Can you work these out from the model? Positions are in its coordinate system, mm. A direction names the side the tool comes from. Round coordinates to 2 decimals unless told otherwise and drop trailing zeros. Order: outer loops, then holes, each group sorted by start corner. A loop starts at its lowest first (then second) coordinate and runs counter-clockwise, first axis right, second up.
from build123d import *

# Parameters (mm, degrees)
SKETCH001_W   = 10
SKETCH001_H   = 10
SKETCH001_W_2 = 8
SKETCH001_H_2 = 8
PAD_DEPTH     = 254
SKETCH002_R   = 2.5
POCKET_DEPTH  = 43.001


with BuildPart() as part:
    # Sketch → Revolution (revolve)
    with BuildSketch(Plane.XZ):
        with BuildLine():
            Line((0, 0), (11, 0))
            ThreePointArc((11, 0), (30.091883, 7.908117), (38, 27))
            Line((38, 27), (37, 27))
            ThreePointArc((10.999947, 1), (29.384758, 8.615205), (37, 27))
            Line((10.999947, 1), (0, 1))
            Line((0, 0), (0, 1))
        make_face()
    revolve(axis=Axis((0, 0, 0), (0, 0, 1)))

    # Sketch001 (on Face5 of Revolution) → Pad (new body)
    with BuildSketch(Plane(origin=(0, 0, 1), x_dir=(-1, 0, 0), z_dir=(0, 0, 1))):
        Rectangle(SKETCH001_W, SKETCH001_H)
        Rectangle(SKETCH001_W_2, SKETCH001_H_2, mode=Mode.SUBTRACT)
    extrude(amount=PAD_DEPTH)

    # Sketch002 (on Face9 of Pad) → Pocket (cut, through all)
    with BuildSketch(Plane(origin=(5, 0, 0), x_dir=(0, 0, 1), z_dir=(1, 0, 0))):
        with Locations((250, 0)):
            Circle(SKETCH002_R)
        with Locations((210, 0)):
            Circle(SKETCH002_R)
    extrude(amount=-POCKET_DEPTH, mode=Mode.SUBTRACT)


solid = part.part
(1) On a 3-axis mill with a long thin cutter (end or side, diameter ignored), from which of +Z, -Z, +X, -X, +Y, -Y can I reach the whole of each face in a straight line? I mean faces 1 (the face through (0, 4, 126)), 2 (the face through (4.5, -0.1, 255)). Say none if no direction works.
(2) I want a section at C-C, the plane y = 0. Give the number of separate pieces and of enclosed holes in the cut face, plus the area to 3 significant figures.
(3) If we mould it in two halves opening along X, with no side actions, what happens to faces 3 (the face through (4, 0, 126)), 4 (the face through (-4.493, -0.751, 252.385))? For each: pulls with the +X half, pulls with the -X half, needs draft (parallel to the pull), parting line crosses it, or undercut.
(4) I'm going to push flat-ended pins straight in: pin 1 Ø24 at (x, y) = (3.5, -3.5) entering from +Z; pin 2 Ø12 at (x, z) = (5.5, 114.5) entering from +Y; pin 3 Ø12 at (y, z) = (3, 206.5) entering from +X; pin 4 Ø2.5 at (x, y) = (-1.5, -1) entering from +Z. Where does each tip first touch, or does it pass through?
(5) I want a section at B-B, the plane z = 47. List the corners of the cut face in (x, y) for me.
(6) Please list where these lines run through material, in increasing order: probe 1 along Z at (x, y) = (-4.65, 0); probe 2 along Y at (x, z) = (-3, 69.5); probe 3 along Y at (x, z) = (-4.75, 250).
(7) I want a section at A-A, the plane z = 250. List the corners of the cut face in (x, y) for me, plus the area to 3 significant figures.
Ans:
1. face 1: +Z
1. face 2: +Z, +X, -X, +Y, -Y
2. separate pieces: 5
2. enclosed holes: 0
2. area: 593 mm2
3. face 3: undercut
3. face 4: needs draft
4. pin 1: stops at z = 255
4. pin 2: stops at y = 5
4. pin 3: stops at x = 5
4. pin 4: stops at z = 1
5. outline: (-5, -5) - (5, -5) - (5, 5) - (-5, 5) - close; hole (-4, -4) - (4, -4) - (4, 4) - (-4, 4) - close
6. probe 1: z = 0 to 207.5, 212.5 to 247.5, 252.5 to 255
6. probe 2: y = -5 to -4, 4 to 5
6. probe 3: y = -5 to -2.5, 2.5 to 5
7. outline: (-5, -5) - (5, -5) - (5, -2.5) - (4, -2.5) - (4, -4) - (-4, -4) - (-4, -2.5) - (-5, -2.5) - close; (-5, 2.5) - (-4, 2.5) - (-4, 4) - (4, 4) - (4, 2.5) - (5, 2.5) - (5, 5) - (-5, 5) - close
7. area: 26.0 mm2
